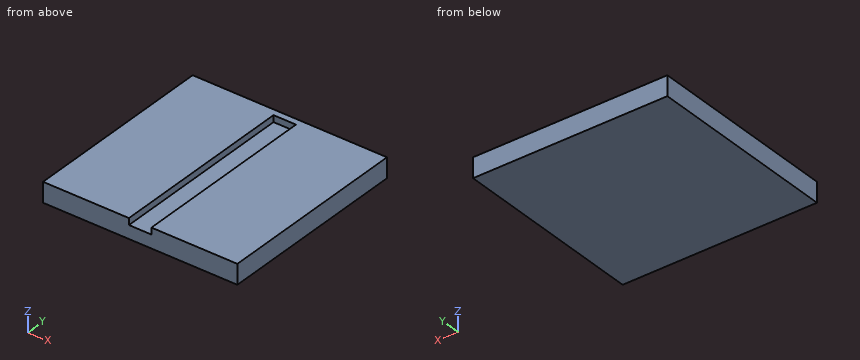
Autodesk Inventor part; units mm, degrees
ref_plane "YZ Plane" through (0, 0, 0) normal (1, 0, 0) x (0, 1, 0)
ref_plane "XZ Plane" through (0, 0, 0) normal (0, 1, 0) x (-1, 0, 0)
ref_plane "XY Plane" through (0, 0, 0) normal (0, 0, 1) x (1, 0, 0)
sketch "Sketch1" plane through (0, 0, 0) normal (0, 0, 1) x (1, 0, 0)
  line L0 (0, 0) -> (14.7, 0)
  line L1 (14.7, 0) -> (14.7, 14.7)
  line L2 (14.7, 14.7) -> (0, 14.7)
  line L3 (0, 14.7) -> (0, 0)
  dimension "d0" = 14.7
  dimension "d1" = 14.7
extrude "Extrusion1" add sketch "Sketch1" along normal blind 1.5
sketch "Sketch2" plane through (0, 0, 1.5) normal (0, 0, 1) x (1, 0, 0)
  line L0 (0, 0) -> (14.7, 0)
  line L1 (14.7, 14.7) -> (0, 14.7)
  line L2 (8.2, 14.7) -> (8.2, 0)
  line L3 (6.5, 14.7) -> (6.5, 0)
  dimension "d6" = 1.7
  dimension "d7" = 6.5
extrude "Extrusion2" cut sketch "Sketch2" against normal blind 0.5
sketch "Sketch3" plane through (0, 0, 1) normal (0, 0, 1) x (1, 0, 0)
  line L0 (8.2, 14.7) -> (8.2, 0)
  line L1 (6.5, 14.7) -> (8.2, 14.7)
  line L2 (8.2, 14.7) -> (8.2, 14.2)
  line L3 (8.2, 14.2) -> (6.5, 14.2)
  line L4 (6.5, 14.2) -> (6.5, 14.7)
  point P0 (0, 0)
  dimension "d8" = 0.5
extrude "Extrusion3" add sketch "Sketch3" along normal blind 0.5
properties part number "Voorplaat"
Geometry: final body of the model. Coordinates: model frame, mm. Give positions to 0.01 mm unless a question says otherwise; leave off trailing zeros. Write each loop counter-clockwise with the first axis right and the second up, starting at its lowest first coordinate (ties: lowest second). Pieces come first, ordered by that corner, then holes.
1. Section query A-A, the plane y = 8.5. Return loops of the section in (x, z).
2. Pin query (flat end, axial travel): P1, Ø0.6, axis at x = 7, z = 1.5, coming from the -Y side; P2, Ø1.9, axis at x = 7.5, y = 7.5, coming from the +Z side. Return the tip coordinate at first contact, or that it passes through.
3. Section query C-C, the plane x = 8. Return loops of the section in (y, z), then the cut area to 4 significant figures.
4. Section query B-B, the plane z = 1.2. Return loops of the section in (x, y).
5. Line query: probe 1 along X at (y, z) = (3, 1.05); probe 2 along Z at (x, y) = (7.75, 13.5). Output: solid intervals per line, ascending.
Computed:
1. outline: (0, 0) - (14.7, 0) - (14.7, 1.5) - (8.2, 1.5) - (8.2, 1) - (6.5, 1) - (6.5, 1.5) - (0, 1.5) - close
2. P1: stops at y = 14.2
2. P2: stops at z = 1.5
3. outline: (0, 0) - (14.7, 0) - (14.7, 1.5) - (14.2, 1.5) - (14.2, 1) - (0, 1) - close
3. area: 14.95 mm2
4. outline: (0, 0) - (6.5, 0) - (6.5, 14.2) - (8.2, 14.2) - (8.2, 0) - (14.7, 0) - (14.7, 14.7) - (0, 14.7) - close
5. probe 1: x = 0 to 6.5, 8.2 to 14.7
5. probe 2: z = 0 to 1
